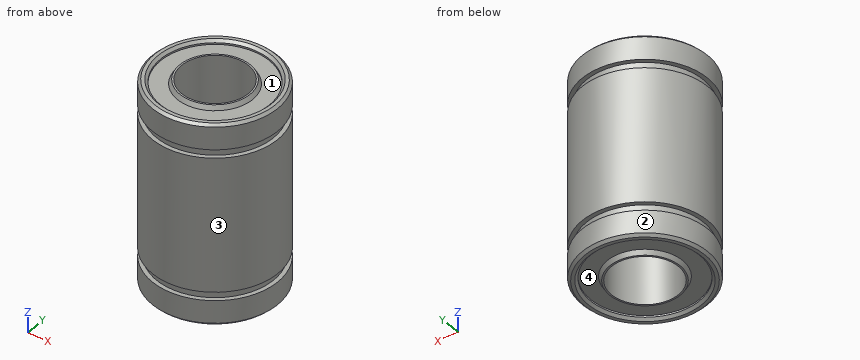
Autodesk Inventor part; units mm, degrees
ref_plane "YZ Plane" through (0, 0, 0) normal (1, 0, 0) x (0, 1, 0)
ref_plane "XZ Plane" through (0, 0, 0) normal (0, 1, 0) x (-1, 0, 0)
ref_plane "XY Plane" through (0, 0, 0) normal (0, 0, 1) x (1, 0, 0)
sketch "Эскиз1" plane through (0, 0, 0) normal (0, 0, 1) x (1, 0, 0)
  circle A0 centre (0, 0) radius 4
  circle A1 centre (0, 0) radius 7.5
  circle A2 centre (0, 0) radius 6.5
  circle A3 centre (0, 0) radius 4.5
  circle A4 centre (0, 0) radius 7
  dimension "d0" = 8
  dimension "d1" = 15
  dimension "d2" = 1
  dimension "d3" = 0.5
  dimension "d25" = 0.5
extrude "Выдавливание1" add sketch "Эскиз1" along normal mid plane 24 contours A3
extrude "Выдавливание2" add sketch "Эскиз1" along normal mid plane 23 contours A2
extrude "Выдавливание3" add sketch "Эскиз1" along normal mid plane 24 contours A1 | A4
chamfer "Фаска1" distance 0.3 angle 45 1 edges at (-6.5, 0, 12)
chamfer "Фаска2" distance 0.3 angle 45 1 edges at (-7.5, 0, 12)
chamfer "Фаска3" distance 0.3 angle 45 2 edges at (-7.5, 0, -12) (-6.5, 0, -12)
chamfer "Фаска4" distance 0.3 distance2 0.5 1 edges at (-4.5, 0, -12) measured on face at (4.251, -0.6781, -12)
chamfer "Фаска5" distance 0.3 distance2 0.5 1 edges at (-4.5, 0, 12) measured on face at (4.251, -0.6781, 12)
extrude "Выдавливание4" cut sketch "Эскиз1" along normal mid plane 18 contours A1
extrude "Выдавливание5" add sketch "Эскиз1" along normal mid plane 16 contours A1
properties part number "линейный подшипник 8х15х24"
Work out the finished part from the listing and answer in its coordinate system (mm). Face numbers are marked on the shaded views. A direction names the side the tool comes from. Give positions to 0.01 mm unless a question says otherwise; leave off trailing zeros. Order: outer loops, then holes, each group sorted by start corner. A loop starts at its lowest first (then second) coordinate and runs counter-clockwise, first axis right, second up. Notation, with made-up numbers: M -18.75,-40 L -4.75,-40 A36 cw -4.75,-6 Z; hole C -19.75,69 d8. An arc over 180 degrees is marked long. Return JSON: item names as keys, results as strings.
Q1. Find the intervals of material crossed by line 1 along Z through (x, y) = (-6.5, 2.75); line 2 along Y through (x, z) = (0, -11.6); line 3 along Y through (x, z) = (0, -0.5), in increasing order. Write a range as [from, to].
Answer below:
{"line 1": "z = [-12, -9], [-8, 8], [9, 12]", "line 2": "y = [-7.5, -6.5], [-4.44, -4], [4, 4.44], [6.5, 7.5]", "line 3": "y = [-7.5, -4], [4, 7.5]"}
Q2. Each of these flat-tipped pins is pushed along its axis until it touches: pin 1 (5 mm diameter, centred on x = 0, y = 0, fed in from -Z); pin 2 (4.5 mm diameter, centred on x = -3.5, y = -1, fed in from +Z); pin 3 (8 mm diameter, centred on y = -4.5, z = -8.5, fed in from -X); pin 4 (6 mm diameter, centred on x = -3.5, z = 4, fed in from -Y). Where does it stop, or does it pass through?
Answer below:
{"pin 1": "passes through", "pin 2": "stops at z = 12", "pin 3": "stops at x = -7.48", "pin 4": "stops at y = -7.48"}
Q3. The mould has two halves that part along Y. Classify the marked faces 1 and 2: pulls with the +Y half, pulls with the -Y half, needs draft (parallel to the pull), parting line crosses it, or undercut.
Answer below:
{"face 1": "undercut", "face 2": "parting line crosses it"}
Q4. Find section A-A, the plane z = 4.75. Write down the section's boundary in (x, y), and give its area (3 significant figures).
Answer below:
{"outline": "C 0,0 d15; hole C 0,0 d8", "area": "126 mm^2"}
Q5. Which of the six approach directions +Z, -Z, +X, -X, +Y, -Y give full straight-line access (tool end or side, diameter ignored) to the marked faces 3 and 4?
Answer below:
{"face 3": "+Z, -Z", "face 4": "-Z"}
